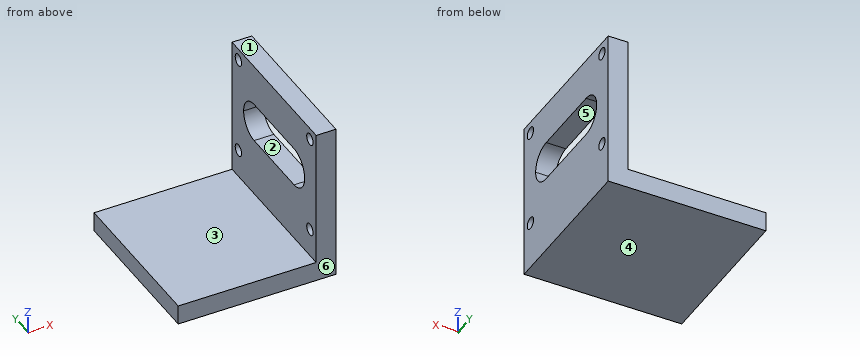
```python
from build123d import *

# Parameters (mm, degrees)
BOSS_EXTRUDE1_DEPTH = 80
SKETCH2_R           = 3
CUT_EXTRUDE1_DEPTH  = 10
CUT_EXTRUDE2_DEPTH  = 10


with BuildPart() as part:
    # Sketch1 → Boss-Extrude1 (new body)
    with BuildSketch(Plane(origin=(0, 0, 0), x_dir=(1, 0, 0), z_dir=(0, 1, 0))):
        Polygon((0, 0), (0, 80.5), (-80, 80.5), (-80, 70.5), (-10, 70.5), (-10, 0), align=None)
    extrude(amount=BOSS_EXTRUDE1_DEPTH)

    # Sketch2 → Cut-Extrude1 (cut)
    with BuildSketch(Plane(origin=(0, 0, 0), x_dir=(0, 0, -1), z_dir=(1, 0, 0))):
        with Locations((6, 6)):
            Circle(SKETCH2_R)
        with Locations((6, 74)):
            Circle(SKETCH2_R)
        with Locations((56, 74)):
            Circle(SKETCH2_R)
        with Locations((56, 6)):
            Circle(SKETCH2_R)
    extrude(amount=-CUT_EXTRUDE1_DEPTH, mode=Mode.SUBTRACT)

    # Sketch3 → Cut-Extrude2 (cut)
    with BuildSketch(Plane(origin=(0, 0, 0), x_dir=(0, 0, -1), z_dir=(1, 0, 0))):
        with BuildLine():
            Line((21, 59), (21, 21))
            ThreePointArc((21, 21), (23.928932188, 13.928932188), (31, 11))
            ThreePointArc((31, 11), (38.071067812, 13.928932188), (41, 21))
            Line((41, 21), (41, 59))
            ThreePointArc((41, 59), (38.071067812, 66.071067812), (31, 69))
            ThreePointArc((31, 69), (23.928932188, 66.071067812), (21, 59))
        make_face()
    extrude(amount=-CUT_EXTRUDE2_DEPTH, mode=Mode.SUBTRACT)


solid = part.part
```
CAD build for the part. Positions are in the model's coordinates, mm. Face numbers are marked on the shaded views. A direction names the side the tool comes from. Coordinates: 2 decimals unless noted, no trailing zeros. Loops run counter-clockwise (first coordinate to the right, second up) from the corner with the lowest first, then second, coordinate; pieces in that order, holes last. Notation, with made-up numbers: (47.25, 18.25) - (74.25, 18.25) arc R19 ccw to (74.25, 23.25) - close; hole circle Ø1 at (6.25, 2.5). An arc over 180 degrees is marked (long way). Return JSON: item names as keys, results as strings.
1. 3-axis set-ups, long thin cutter, end or side, ignore diameter. For the marked faces 1, 2 and 3: which of +Z, -Z, +X, -X, +Y, -Y reach the whole face in a straight line?
Result:
{"face 1": "+Z, +X, -X, +Y, -Y", "face 2": "+X, -X", "face 3": "+Z, -X, +Y, -Y"}
2. Drop flat-ended pins along their axis: pin 1 (5.5 mm diameter, centred on y = 74, z = -6, fed in from +X); pin 2 (8 mm diameter, centred on y = 66, z = -28.5, fed in from -X). Give the stop position or say it passes through.
Result:
{"pin 1": "passes through", "pin 2": "stops at x = -10"}
3. Probe L1, parallel to Y at x = -4, z = -56; L2, parallel to Z at x = -35.5, y = 43; L3, parallel to X at y = 10, z = -48. List the from-to ranges inside material, lowest first. Write a range as from..to.
Result:
{"L1": "y = 0..3, 9..71, 77..80", "L2": "z = -80.5..-70.5", "L3": "x = -10..0"}
4. Mould opens along Y. For the marked faces 4, 5 and 6 say: released by +Y, released by -Y, zero draft, split by the parting line, or undercut.
Result:
{"face 4": "zero draft", "face 5": "undercut", "face 6": "released by -Y"}
5. Band-saw the part on D-D (z = -34.5). Give the cut face in (x, y), and give its area (3 significant figures).
Result:
{"outline": "(-10, 0) - (0, 0) - (0, 11.63) - (-10, 11.63) - close; (-10, 68.37) - (0, 68.37) - (0, 80) - (-10, 80) - close", "area": "233 mm2"}
6. Band-saw the part on B-B (y = 27). Give the cut face in (x, z), and give its area (4 significant figures).
Result:
{"outline": "(-80, -80.5) - (0, -80.5) - (0, -41) - (-10, -41) - (-10, -70.5) - (-80, -70.5) - close; (-10, -21) - (0, -21) - (0, 0) - (-10, 0) - close", "area": "1,305 mm2"}
7. Band-saw the part on A-A (z = -6). Give the cut face in (x, y), and give its area (3 significant figures).
Result:
{"outline": "(-10, 0) - (0, 0) - (0, 3) - (-10, 3) - close; (-10, 9) - (0, 9) - (0, 71) - (-10, 71) - close; (-10, 77) - (0, 77) - (0, 80) - (-10, 80) - close", "area": "680 mm2"}
8. Band-saw the part on C-C (y = 6). Give the cut face in (x, z).
Result:
{"outline": "(-80, -80.5) - (0, -80.5) - (0, -59) - (-10, -59) - (-10, -70.5) - (-80, -70.5) - close; (-10, -53) - (0, -53) - (0, -9) - (-10, -9) - close; (-10, -3) - (0, -3) - (0, 0) - (-10, 0) - close"}
